CAD build for the part. Positions are in the model's coordinates, mm. Give positions to 0.01 mm unless a question says otherwise; leave off trailing zeros. Order: outer loops, then holes, each group sorted by start corner. A loop starts at its lowest first (then second) coordinate and runs counter-clockwise, first axis right, second up.
Item 1: Two-plate mould, pull along X, no slides. Class faces 1 (the cylindrical face through (-2.648, 11.927, 197.028)), 2 (the flat face through (12.34, 1.16, 401.16)), 3 (the cylindrical face through (-3.634, 16.365, 196.965)): released by +X, released by -X, zero draft, split by the parting line, or undercut.
Item 2: Band-saw the part on C-C on z = 146. Give the cut face in (x, y), plus the area to 3 significant figures.
Item 3: Band-saw the part on B-B on x = -7. Give the cut face in (y, z), plus the area to 3 significant figures.
Item 4: Band-saw the part on A-A on y = 0. Give the cut face in (x, z).
Item 5: Wall check: L1, parallel to X at y = -1, z = 194.5; L2, parallel to Y at x = 0, z = 190. Give the ranges that are in metal, low to high.
Item 6: Flat gauge pins, fed straight in: P1, Ø12, axis at x = 9, y = 12.5, coming from the -Z side; P2, Ø5, axis at y = -8.5, z = 227, coming from the +X side; P3, Ø1.5, axis at x = -13, z = 127, coming from the +Y side. Where does each tip first touch, or does it go through?
Autodesk Inventor part; units mm, degrees
ref_plane "Start Plane" through (0, 0, -16.764) normal (0, 0, 1) x (1, 0, 0)
ref_plane "End Plane" through (0, 0, 416.764) normal (0, 0, 1) x (1, 0, 0)
ref_plane "Work Plane4" through (0, 16.764, 416.764) normal (0, -0.7071, 0.7071) x (1, 0, 0)
ref_plane "Start Plane" through (0, 0, -16.764) normal (0, 0, 1) x (1, 0, 0)
ref_plane "End Plane" through (0, 0, 416.764) normal (0, 0, 1) x (1, 0, 0)
sketch "Sketch" plane through (0, 0, 0) normal (0, 0, 1) x (1, 0, 0)
  circle A0 centre (0, 0) radius 12.2174
  circle A1 centre (0, 0) radius 16.764
  dimension "d0" = 33.528
  dimension "d1" = 4.5466
extrude "Body" add sketch "Sketch" along normal up to surface (433.528 mm away) from surface at -16.764
sketch "Sketch3" plane through (0, 0, 0) normal (0, 0, 1) x (1, 0, 0)
  line L0 (0, 0) -> (10, 0)
ref_plane "Work Plane3" through (0, 0, 0) normal (0, -1, 0) x (1, 0, 0)
ref_plane "Work Plane4" through (0, 16.764, 416.764) normal (0, -0.7071, 0.7071) x (1, 0, 0)
split "Split1" plane through (0, 16.764, 416.764) removes the side toward (0, -0.7071, 0.7071)
ref_plane "Work Plane5" through (0, 16.764, -16.764) normal (0, -0.7071, -0.7071) x (1, 0, 0)
split "Split2" plane through (0, 16.764, -16.764) removes the side toward (0, -0.7071, -0.7071)
sketch "Sketch4" plane through (0, 0, 0) normal (0, -1, 0) x (1, 0, 0)
  line L0 (-2, -16.764) -> (12, -16.764)
  line L1 (-2, 416.764) -> (12, 416.764)
  dimension "d7" = 433.528
equation "\"d0\" = G_H"
equation "\"d1\" = G_T"
equation "\"d2\" = G_L"
equation "\"G_H\" = 33.528"
equation "\"G_T\" = 4.5466"
equation "\"G_L\" = d7"
equation "\"G_OFFSET_START\" = 16.764"
equation "\"G_OFFSET_END\" = 16.764"
equation "\"d4\" = -G_OFFSET_START"
equation "\"d5\" = G_OFFSET_END + B_L"
equation "\"B_L\" = 400"
properties part number "ANSI - 1 x 0.179 - 17.068" material "Steel, Mild"
The answers:
1. face 1: undercut
1. face 2: zero draft
1. face 3: split by the parting line
2. outline: circle Ø33.53 at (0, 0); hole circle Ø24.43 at (0, 0)
2. area: 414 mm2
3. outline: (-15.23, 15.23) - (-10.01, 10.01) - (-10.01, 389.99) - (-15.23, 384.77) - close; (10.01, -10.01) - (15.23, -15.23) - (15.23, 415.23) - (10.01, 410.01) - close
3. area: 4,180 mm2
4. outline: (-16.76, 0) - (-12.22, 0) - (-12.22, 400) - (-16.76, 400) - close; (12.22, 0) - (16.76, 0) - (16.76, 400) - (12.22, 400) - close
5. L1: x = -16.73 to -12.18, 12.18 to 16.73
5. L2: y = -16.76 to -12.22, 12.22 to 16.76
6. P1: stops at z = -16.21
6. P2: stops at x = 15.65
6. P3: stops at y = 11.44
